Drawing for the job (mm, zero at the part's lowest x, y, z). Round coordinates to 2 decimals unless told otherwise and drop trailing zeros. Write each loop counter-clockwise with the first axis right and the second up, starting at its lowest first coordinate (ties: lowest second). Pieces come first, ordered by that corner, then holes. Notation, with made-up numbers: (-17, -28) -> (-5, -28) arc R33 ccw to (-5, 4) -> close; hole circle Ø9 at (-0.75, 12). An arc over 180 degrees is marked (long way). One line per question, with ' | ' between items.
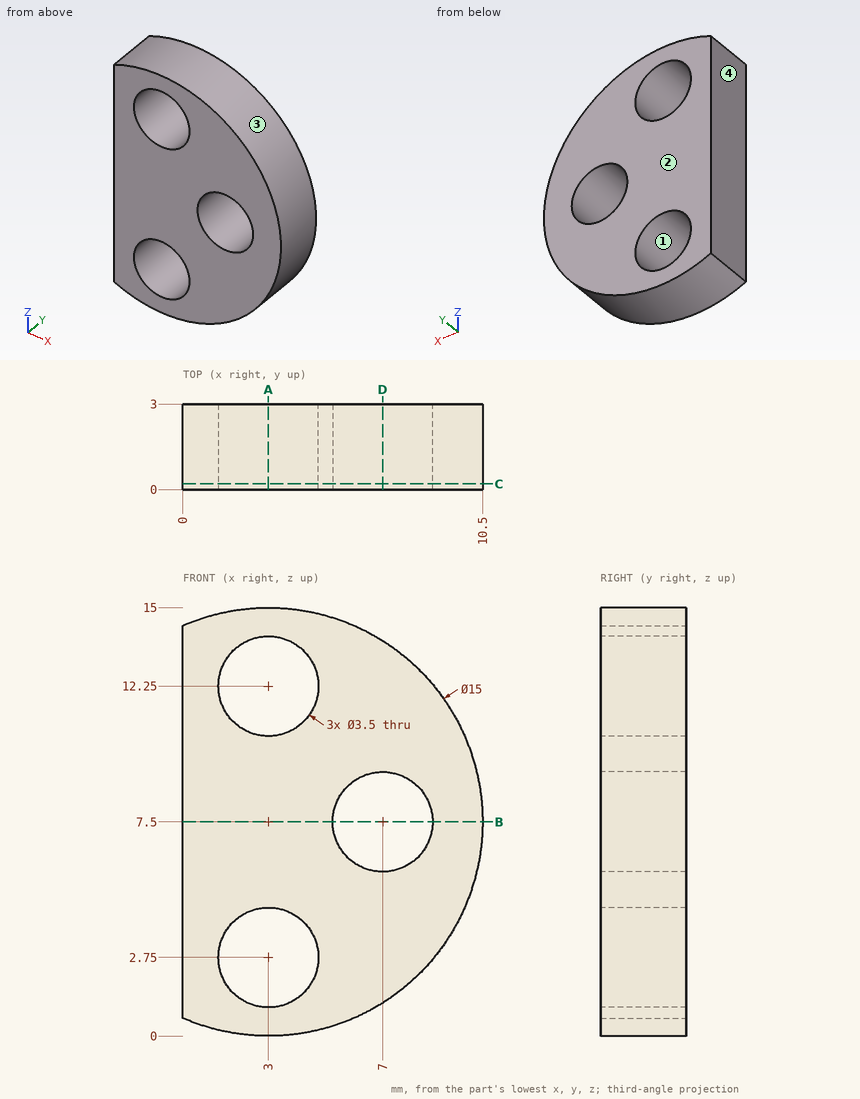
(1) Slice it at B-B (z = 7.5). Write the cut outline in (x, y).
Calculated:
outline: (0, 0) -> (5.25, 0) -> (5.25, 3) -> (0, 3) -> close; (8.75, 0) -> (10.5, 0) -> (10.5, 3) -> (8.75, 3) -> close
(2) Slice it at D-D (x = 7). Write the cut outline in (y, z), then the cut area to 3 significant figures.
Calculated:
outline: (0, 1.16) -> (3, 1.16) -> (3, 5.75) -> (0, 5.75) -> close; (0, 9.25) -> (3, 9.25) -> (3, 13.84) -> (0, 13.84) -> close | area: 27.6 mm2
(3) Slice it at C-C (y = 0.2). Write the cut outline in (x, z), then the cut area to 3 significant figures.
Calculated:
outline: (0, 0.63) arc R7.5 ccw (long way) to (0, 14.37) -> close; hole circle Ø3.5 at (3, 2.75); hole circle Ø3.5 at (3, 12.25); hole circle Ø3.5 at (7, 7.5) | area: 103 mm2
(4) Wall check: line 1 (Z direction, x = 3, y = 1.45); line 2 (X direction, y = 2.15, z = 7.5); line 3 (X direction, y = 2.85, z = 3). Give the ranges that are in metal, low to high. Write a range as from..to.
Calculated:
line 1: 0..1, 4.5..10.5, 14..15 | line 2: 0..5.25, 8.75..10.5 | line 3: 0..1.27, 4.73..9
(5) Slice it at A-A (x = 3). Write the cut outline in (y, z), then the cut area to 3 significant figures.
Calculated:
outline: (0, 0) -> (3, 0) -> (3, 1) -> (0, 1) -> close; (0, 4.5) -> (3, 4.5) -> (3, 10.5) -> (0, 10.5) -> close; (0, 14) -> (3, 14) -> (3, 15) -> (0, 15) -> close | area: 24.0 mm2
(6) Mould opens along X. For the marked faces 1, 2, 3 and 4 say: pulls with the +X half, pulls with the -X half, needs draft (parallel to the pull), parting line crosses it, or undercut.
Calculated:
face 1: undercut | face 2: needs draft | face 3: parting line crosses it | face 4: pulls with the -X half
